```python
from build123d import *

# Parameters (mm, degrees)
SKETCH1_W           = 28
SKETCH1_H           = 22
BOSS_EXTRUDE1_DEPTH = 10
SKETCH5_W           = 7
SKETCH5_H           = 7
CUT_EXTRUDE7_DEPTH  = 22
SKETCH2_R           = 11
CUT_EXTRUDE8_DEPTH  = 7
SKETCH6_R           = 7
CUT_EXTRUDE9_DEPTH  = 3
SKETCH7_R           = 1.5
CUT_EXTRUDE10_DEPTH = 10


with BuildPart() as part:
    # Sketch1 → Boss-Extrude1 (new body)
    with BuildSketch(Plane(origin=(0, 0, 0), x_dir=(1, 0, 0), z_dir=(0, 1, 0))):
        Rectangle(SKETCH1_W, SKETCH1_H)
    extrude(amount=BOSS_EXTRUDE1_DEPTH)

    # Sketch5 → Cut-Extrude7 (cut)
    with BuildSketch(Plane(origin=(0, 0, -11), x_dir=(-1, 0, 0), z_dir=(0, 0, -1))):
        with Locations((0, 6.5)):
            Rectangle(SKETCH5_W, SKETCH5_H)
    extrude(amount=-CUT_EXTRUDE7_DEPTH, mode=Mode.SUBTRACT)

    # Sketch2 → Cut-Extrude8 (cut)
    with BuildSketch(Plane(origin=(0, 10, 0), x_dir=(1, 0, 0), z_dir=(0, 1, 0))):
        Circle(SKETCH2_R)
    extrude(amount=-CUT_EXTRUDE8_DEPTH, mode=Mode.SUBTRACT)

    # Sketch6 → Cut-Extrude9 (cut)
    with BuildSketch(Plane.XZ):
        with Locations(Location((0, 0, 0), (0, 0, 270))):
            Circle(SKETCH6_R)
    extrude(amount=-CUT_EXTRUDE9_DEPTH, mode=Mode.SUBTRACT)

    # Sketch7 → Cut-Extrude10 (cut)
    with BuildSketch(Plane.XZ):
        with Locations(Location((11, 8, 0), (0, 0, 270))):
            Circle(SKETCH7_R)
        with Locations(Location((11, -8, 0), (0, 0, 90))):
            Circle(SKETCH7_R)
        with Locations(Location((-11, -8, 0), (0, 0, 270))):
            Circle(SKETCH7_R)
        with Locations(Location((-11, 8, 0), (0, 0, 90))):
            Circle(SKETCH7_R)
    extrude(amount=-CUT_EXTRUDE10_DEPTH, mode=Mode.SUBTRACT)


solid = part.part
```
Input: part model. Units: mm. Frame: model coordinates. A direction names the side the tool comes from. Round coordinates to 2 decimals unless told otherwise and drop trailing zeros. Loops run counter-clockwise (first coordinate to the right, second up) from the corner with the lowest first, then second, coordinate; pieces in that order, holes last. Notation, with made-up numbers: (-36.5, 81.5) - (-11.5, 81.5) arc R33 cw to (-11.5, 112.5) - close; hole circle Ø8 at (18, -5). An arc over 180 degrees is marked (long way). One line per item, written item: value. Start each with the question number.
(1) Section A-A, the plane y = 4. Return loops of the section in (x, z).
(2) Section B-B, the plane z = 0. Return loops of the section in (x, y), plus the area to 3 significant figures.
(3) Access query for faces 1 (the flat face through (14, 5, 0)), 2 (the cylindrical face through (11, 7, 0)). Directions: +Z, -Z, +X, -X, +Y, -Y. A direction counts if a zero-diameter tool reaches every point of the face in a straight line with its end or side. Return the directions, or none.
(4) Ray query, line 1 (X direction, y = 0.6, z = 0); line 2 (X direction, y = 2, z = 8); line 3 (X direction, y = 3.5, z = 8). Return the intervals inside material, ascending. Write a range as [from, to].
(5) Draft query along Z for faces 3 (the flat face through (0.2, 3, 7.2)), 4 (the flat face through (-0.2, 2.7, -11)), 5 (the cylindrical face through (-11, 7, 0)), 6 (the flat face through (-0.2, 0, -7.5)). Return one class per face: +Z half, -Z half, draft (parallel to the pull), parting line (faces both ways), or undercut.
(6) Contact query for flat-ended pins moving along their axis: P1, Ø1.8, axis at x = -11, z = -8, coming from the +Y side; P2, Ø6, axis at x = -3, z = -3.5, coming from the +Y side. Output: stop coordinate, or through.
(7) Section C-C, the plane x = 12. Return loops of the section in (y, z).
(8) Section D-D, the plane z = -8. Return loops of the section in (x, y).
Results below:
1. outline: (-14, -11) - (-3.5, -11) - (-3.5, -10.43) arc R11 cw to (-3.5, 10.43) - (-3.5, 11) - (-14, 11) - close; (3.5, -11) - (14, -11) - (14, 11) - (3.5, 11) - (3.5, 10.43) arc R11 cw to (3.5, -10.43) - close; hole circle Ø3 at (-11, -8); hole circle Ø3 at (-11, 8); hole circle Ø3 at (11, -8); hole circle Ø3 at (11, 8)
2. outline: (-14, 0) - (-7, 0) - (-7, 3) - (-11, 3) - (-11, 10) - (-14, 10) - close; (7, 0) - (14, 0) - (14, 10) - (11, 10) - (11, 3) - (7, 3) - close
2. area: 84.0 mm^2
3. face 1: +Z, -Z, +X, +Y, -Y
3. face 2: +Y
4. line 1: [-14, -7], [7, 14]
4. line 2: [-14, -12.5], [-9.5, 9.5], [12.5, 14]
4. line 3: [-14, -12.5], [-9.5, -7.55], [7.55, 9.5], [12.5, 14]
5. face 3: undercut
5. face 4: -Z half
5. face 5: undercut
5. face 6: draft
6. P1: through
6. P2: y = 3
7. outline: (0, -11) - (10, -11) - (10, -9.12) - (0, -9.12) - close; (0, -6.88) - (10, -6.88) - (10, 6.88) - (0, 6.88) - close; (0, 9.12) - (10, 9.12) - (10, 11) - (0, 11) - close
8. outline: (-14, 0) - (-12.5, 0) - (-12.5, 10) - (-14, 10) - close; (-9.5, 0) - (9.5, 0) - (9.5, 10) - (7.55, 10) - (7.55, 3) - (-7.55, 3) - (-7.55, 10) - (-9.5, 10) - close; (12.5, 0) - (14, 0) - (14, 10) - (12.5, 10) - close
